from build123d import *

# Parameters (mm, degrees)
SKETCH1_W                = 123
SKETCH1_H                = 123
SKETCH1_R                = 46
BOSS_EXTRUDE1_DEPTH      = 2
FILLET1_R                = 5
M2_CLEARANCE_HOLE1_D     = 2.4
M2_CLEARANCE_HOLE1_DEPTH = 4


with BuildPart() as part:
    # Sketch1 → Boss-Extrude1 (new body, symmetric)
    with BuildSketch(Plane.XY):
        Rectangle(SKETCH1_W, SKETCH1_H)
        Circle(SKETCH1_R, mode=Mode.SUBTRACT)
    extrude(amount=BOSS_EXTRUDE1_DEPTH, both=True)

    # Fillet1
    fillet1_edges = [part.edges().sort_by_distance(p)[0] for p in [
        (-61.5, -61.5, 0),
        (-61.5, 61.5, 0),
        (61.5, 61.5, 0),
        (61.5, -61.5, 0),
    ]]
    fillet(fillet1_edges, radius=FILLET1_R)

    # M2 Clearance Hole1
    with Locations(Plane.XY.offset(2)):
        with Locations((58.5, -18.833333333), (-57.914213562, 57.914213562), (57.914213562, 57.914213562), (57.914213562, -57.914213562), (-57.914213562, -57.914213562), (-18.833333333, -58.5), (18.833333333, -58.5), (-58.5, -18.833333333), (-58.5, 18.833333333), (-18.833333333, 58.5), (18.833333333, 58.5), (58.5, 18.833333333)):
            Hole(M2_CLEARANCE_HOLE1_D / 2, depth=M2_CLEARANCE_HOLE1_DEPTH)


solid = part.part
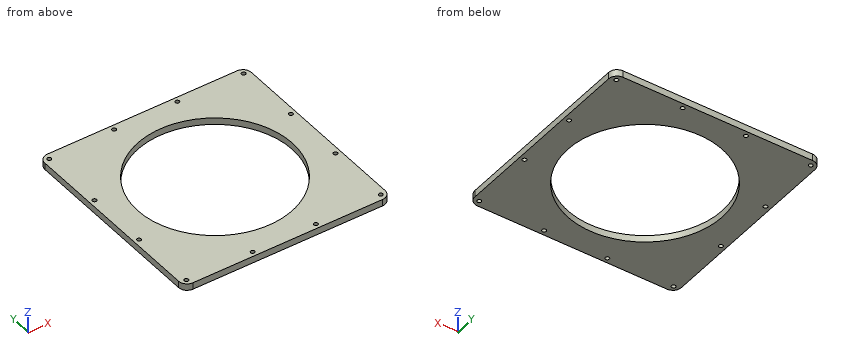
The listing builds one solid part. Answer for the finished solid, in the listing's coordinates (mm). Coordinates: 2 decimals unless noted, no trailing zeros. Write each loop counter-clockwise with the first axis right and the second up, starting at its lowest first coordinate (ties: lowest second). Pieces come first, ordered by that corner, then holes. Notation, with made-up numbers: (73.5, 25) - (99.5, 25) arc R32 ccw to (99.5, 52) - close; hole circle Ø4 at (14.25, 1). An arc over 180 degrees is marked (long way). Return JSON: item names as keys, results as strings.
1. The part is cut by section A-A on x = 0. Determine the outline of the cut face in (y, z), then the cut area to 3 significant figures.
Final values:
{"outline": "(-61.5, -2) - (-46, -2) - (-46, 2) - (-61.5, 2) - close; (46, -2) - (61.5, -2) - (61.5, 2) - (46, 2) - close", "area": "124 mm^2"}
2. Consider line 1 along Y through (x, z) = (-58.5, -0.45); line 2 along X through (y, z) = (-29.5, -1.65); line 3 along Y through (x, z) = (9, -0.4). Determine where each line is inside the solid, lowest interval first.
Final values:
{"line 1": "-61.08 to -58.96, -56.87 to -20.03, -17.63 to 17.63, 20.03 to 56.87, 58.96 to 61.08", "line 2": "-61.5 to -35.3, 35.3 to 61.5", "line 3": "-61.5 to -45.11, 45.11 to 61.5"}
3. This flat-tipped pin is pushed along its axis until it touches: pin 1 Ø3 at (x, y) = (-18.83, 58.5) entering from -Z. Where does it stop, or does it pass through?
Final values:
{"pin 1": "z = -2"}
4. The part is cut by section C-C on z = -1.15. Count the separate pieces of the cut face and the enclosed holes in it, then the cut area to 3 significant figures.
Final values:
{"separate pieces": "1", "enclosed holes": "13", "area": "8,410 mm^2"}
